from build123d import *

# Parameters (mm, degrees)
ESQUISSE1_W                = 100
ESQUISSE1_H                = 50
BOSS_EXTRU_1_DEPTH         = 10
ESQUISSE2_W                = 10
ESQUISSE2_H                = 10
ENL_V_MAT_EXTRU_1_DEPTH    = 10
R_P_TITION_LIN_AIRE1_COUNT = 5
R_P_TITION_LIN_AIRE1_PITCH = 20


with BuildPart() as part:
    # Esquisse1 → Boss.-Extru.1 (new body)
    with BuildSketch(Plane(origin=(0, 0, 0), x_dir=(0, 0, -1), z_dir=(1, 0, 0))):
        with Locations((-50, 25)):
            Rectangle(ESQUISSE1_W, ESQUISSE1_H)
    extrude(amount=BOSS_EXTRU_1_DEPTH)

    # Esquisse2 → Enlèv. mat.-Extru.1 (cut)
    with BuildSketch(Plane(origin=(10, 0, 0), x_dir=(0, 0, -1), z_dir=(1, 0, 0))):
        with Locations((-15, 45)):
            Rectangle(ESQUISSE2_W, ESQUISSE2_H)
    enl_v_mat_extru_1 = extrude(amount=-ENL_V_MAT_EXTRU_1_DEPTH, mode=Mode.SUBTRACT)

    # Répétition linéaire1: Enlèv. mat.-Extru.1 ×5
    with Locations(*[(0, 0, i * R_P_TITION_LIN_AIRE1_PITCH) for i in range(1, R_P_TITION_LIN_AIRE1_COUNT)]):
        add(enl_v_mat_extru_1, mode=Mode.SUBTRACT)


solid = part.part
Verification items for the finished model (mm, model axes). A direction names the side the tool comes from. Give positions to 0.01 mm unless a question says otherwise; leave off trailing zeros. Order: outer loops, then holes, each group sorted by start corner. A loop starts at its lowest first (then second) coordinate and runs counter-clockwise, first axis right, second up. Notation, with made-up numbers: (60, 88) -> (77, 88) arc R7 ccw to (77, 96) -> close; hole circle Ø3 at (55, 47.25). An arc over 180 degrees is marked (long way). Answer as CSV lines item,"result".
Q1. Sectioned sample at C-C on z = 53. Record the cut outline in (x, y), plus the area to 3 significant figures.
Solutions:
outline,"(0, 0) -> (10, 0) -> (10, 40) -> (0, 40) -> close"
area,"400 mm²"
Q2. Access from +Z, -Z, +X, -X, +Y, -Y to the whole of each face (thin tool, end or side, straight path). Record for faces 4 (the flat face through (5, 40, 95)), 5 (the flat face through (5, 45, 10)), 6 (the flat face through (5, 0, 51)).
Solutions:
face 4,"+Z, +X, -X, +Y"
face 5,"+X, -X, +Y"
face 6,"+Z, -Z, +X, -X, -Y"
Q3. Release check for a two-part mould opening along Z. For faces 1 (the flat face through (5, 20, 100)), 2 (the flat face through (5, 45, 50)), 3 (the flat face through (10, 25, 51)) record: +Z half, -Z half, draft (parallel to the pull), parting line (faces both ways), or undercut.
Solutions:
face 1,"+Z half"
face 2,"undercut"
face 3,"draft"
Q4. Sectioned sample at A-A on y = 41. Record the cut outline in (x, z), plus the area to 3 significant figures.
Solutions:
outline,"(0, 0) -> (10, 0) -> (10, 10) -> (0, 10) -> close; (0, 20) -> (10, 20) -> (10, 30) -> (0, 30) -> close; (0, 40) -> (10, 40) -> (10, 50) -> (0, 50) -> close; (0, 60) -> (10, 60) -> (10, 70) -> (0, 70) -> close; (0, 80) -> (10, 80) -> (10, 90) -> (0, 90) -> close"
area,"500 mm²"
Q5. Sectioned sample at B-B on x = 1.5. Record the cut outline in (y, z), plus the area to 3 significant figures.
Solutions:
outline,"(0, 0) -> (50, 0) -> (50, 10) -> (40, 10) -> (40, 20) -> (50, 20) -> (50, 30) -> (40, 30) -> (40, 40) -> (50, 40) -> (50, 50) -> (40, 50) -> (40, 60) -> (50, 60) -> (50, 70) -> (40, 70) -> (40, 80) -> (50, 80) -> (50, 90) -> (40, 90) -> (40, 100) -> (0, 100) -> close"
area,"4,500 mm²"
Q6. Depth check by flat-ended pin: pin 1 (5 mm diameter, centred on x = 7.5, y = 46, fed in from +Z); pin 2 (3 mm diameter, centred on x = 5, z = 33, fed in from +Y). Enter the tip coordinate at first touch or a pass-through.
Solutions:
pin 1,"stops at z = 90"
pin 2,"stops at y = 40"
Q7. Scan line: probe 1 along Y at (x, z) = (7.25, 77). Record every from-to range of solid material in increasing order.
Solutions:
probe 1,"y = 0 to 40"
